Work out the finished part from the listing and answer in its coordinate system (mm). Face numbers are marked on the shaded views. Round coordinates to 2 decimals unless told otherwise and drop trailing zeros. Write each loop counter-clockwise with the first axis right and the second up, starting at its lowest first coordinate (ties: lowest second). Pieces come first, ordered by that corner, then holes.
1. Find section B-B (y = 0). Write down the section's boundary in (x, z).
2. Find section A-A (x = 0). Write down the section's boundary in (y, z).
3. Determine the mould class of the marked faces 1, 2 and 3 for opening direction X: pulls with the +X half, pulls with the -X half, needs draft (parallel to the pull), parting line crosses it, or undercut.
4. Straight lines are drawn through the part: probe 1 along Y at (x, z) = (0, 0.9); probe 2 along Y at (x, z) = (-7.5, 1.5); probe 3 along X at (y, z) = (-21, 6.25). For each, find the intervals that lie inside material, in ascending order.
5. Find section D-D (x = 10.5). Write down the section's boundary in (y, z), and give its area (3 significant figures).
6. Flat-ended cylindrical pins translate along their axes: pin 1 Ø1 at (x, z) = (10.5, 1) entering from +Y; pin 2 Ø4 at (x, z) = (8.5, 5) entering from -Y; pin 3 Ø3 at (y, z) = (13, 3) entering from +X. Find the tip coordinate at first contact, or state that the pin passes through.
Autodesk Fusion 360 part; units mm, degrees
sketch "Sketch1" plane through (0, 0, 0) normal (0, 0, 1) x (1, 0, 0)
  circle A0 centre (0, 0) radius 27
  circle A1 centre (0, 0) radius 29
  dimension "d1" = 54
  dimension "d2" = 58
extrude "Extrude1" add sketch "Sketch1" along normal blind 3.5
sketch "Sketch2" plane through (0, 0, 0) normal (0, 0, -1) x (1, 0, 0)
  circle A0 centre (0, 0) radius 27
  circle A1 centre (0, 0) radius 29
  circle A2 centre (0, 0) radius 30.5
  dimension "d5" = 61
extrude "Extrude2" add sketch "Sketch2" against normal blind 7 contours A2
sketch "Sketch3" plane through (0, 0, 7) normal (0, 0, 1) x (-1, 0, 0)
  circle A0 centre (0, 0) radius 29
  circle A1 centre (0, 0) radius 30.5
  line L0 (0, 29.5) -> (-6, 29.5) construction
  line L1 (0, 26) -> (0, 34.5) construction
  line L2 (0, 29.5) -> (6, 29.5) construction
  line L3 (5.7478, 28.4247) -> (6.0905, 29.8857)
  line L4 (-5.7478, 28.4247) -> (-6.0905, 29.8857)
  line L5 (-6, 0) -> (15.5156, 0) construction
  line L6 (5.7478, -28.4247) -> (6.0905, -29.8857)
  line L7 (-5.7478, -28.4247) -> (-6.0905, -29.8857)
  dimension "d8" = 6
extrude "Extrude3" cut sketch "Sketch3" against normal blind 3.5 contours A0 A1 L3 L4
extrude "Extrude4" cut sketch "Sketch3" against normal blind 3.5 contours A0 A1 L6 L7
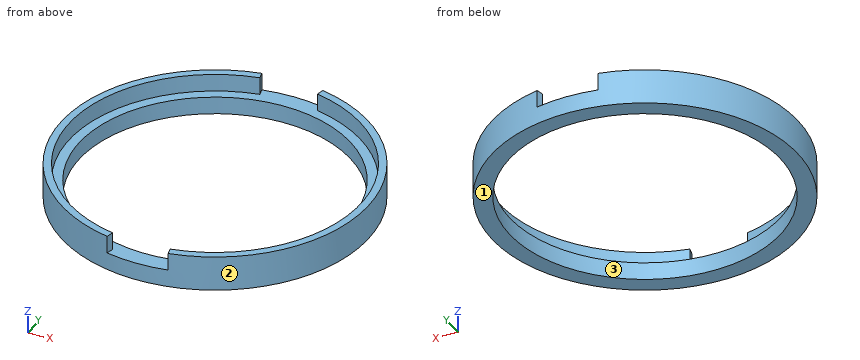
Worked answers:
1. outline: (-30.5, 0) - (-27, 0) - (-27, 3.5) - (-29, 3.5) - (-29, 7) - (-30.5, 7) - close; (27, 0) - (30.5, 0) - (30.5, 7) - (29, 7) - (29, 3.5) - (27, 3.5) - close
2. outline: (-30.5, 0) - (-27, 0) - (-27, 3.5) - (-30.5, 3.5) - close; (27, 0) - (30.5, 0) - (30.5, 3.5) - (27, 3.5) - close
3. face 1: needs draft
3. face 2: parting line crosses it
3. face 3: undercut
4. probe 1: y = -30.5 to -27, 27 to 30.5
4. probe 2: y = -29.56 to -25.94, 25.94 to 29.56
4. probe 3: x = -22.12 to -20, 20 to 22.12
5. outline: (-28.64, 0) - (-24.87, 0) - (-24.87, 3.5) - (-27.03, 3.5) - (-27.03, 7) - (-28.64, 7) - close; (24.87, 0) - (28.64, 0) - (28.64, 7) - (27.03, 7) - (27.03, 3.5) - (24.87, 3.5) - close
5. area: 37.5 mm2
6. pin 1: stops at y = 28.81
6. pin 2: stops at y = -29.8
6. pin 3: stops at x = 28.25
